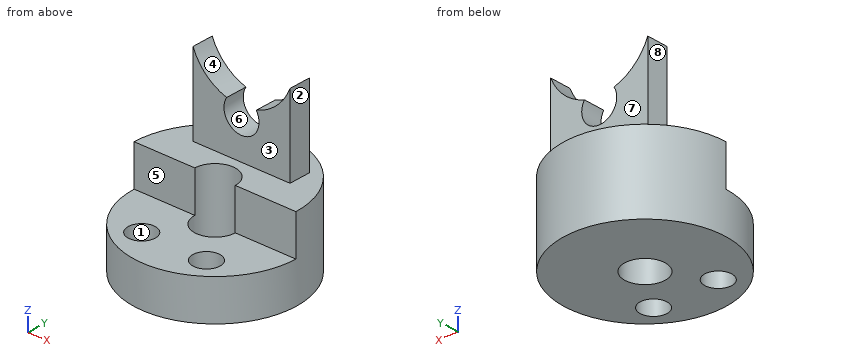
from build123d import *

# Parameters (mm, degrees)
SKETCH_1_R          = 30
EXTRUDE_1_DEPTH     = 15
EXTRUDE_2_DEPTH     = 15
SKETCH_3_R          = 7.5
CUT_EXTRUDE_1_DEPTH = 52.961524227
SKETCH_4_W          = 36
SKETCH_4_H          = 8
EXTRUDE_3_DEPTH     = 30
SKETCH_6_R          = 6.5
CUT_EXTRUDE_3_DEPTH = 79.619336044
SKETCH_5_R          = 19.313207916
CUT_EXTRUDE_4_DEPTH = 79.619336044
SKETCH_7_R          = 5
CUT_EXTRUDE_5_DEPTH = 62.846584384


with BuildPart() as part:
    # Эскиз1 → Бобышка-Вытянуть1 (new body)
    with BuildSketch(Plane.XY):
        Circle(SKETCH_1_R)
    extrude(amount=EXTRUDE_1_DEPTH)

    # Эскиз2 → Бобышка-Вытянуть2 (add)
    with BuildSketch(Plane.XY.offset(15)):
        with BuildLine():
            Line((-30, 0), (30, 0))
            ThreePointArc((30, 0), (0, 30), (-30, 0))
        make_face()
    extrude(amount=EXTRUDE_2_DEPTH)

    # Эскиз3 → Вырез-Вытянуть1 (cut, through all)
    with BuildSketch(Plane.XY.offset(30)):
        Circle(SKETCH_3_R)
    extrude(amount=-CUT_EXTRUDE_1_DEPTH, mode=Mode.SUBTRACT)

    # Эскиз4 → Бобышка-Вытянуть3 (add)
    with BuildSketch(Plane.XY.offset(30)):
        with Locations((0, 15)):
            Rectangle(SKETCH_4_W, SKETCH_4_H)
    extrude(amount=EXTRUDE_3_DEPTH)

    # Эскиз6 → Вырез-Вытянуть3 (cut, through all)
    with BuildSketch(Plane(origin=(0, 11, 0), x_dir=(-1, 0, 0), z_dir=(0, -1, 0))):
        with Locations(Location((0, -45, 0), (0, 0, 90))):
            Circle(SKETCH_6_R)
    extrude(amount=-CUT_EXTRUDE_3_DEPTH, mode=Mode.SUBTRACT)

    # Эскиз5 → Вырез-Вытянуть4 (cut, through all)
    with BuildSketch(Plane(origin=(0, 11, 0), x_dir=(-1, 0, 0), z_dir=(0, -1, 0))):
        with Locations((0, -67)):
            Circle(SKETCH_5_R)
    extrude(amount=-CUT_EXTRUDE_4_DEPTH, mode=Mode.SUBTRACT)

    # Эскиз7 → Вырез-Вытянуть5 (cut, through all)
    with BuildSketch(Plane.XY.offset(15)):
        with Locations((-12, -17)):
            Circle(SKETCH_7_R)
        with Locations((12, -17)):
            Circle(SKETCH_7_R)
    extrude(amount=-CUT_EXTRUDE_5_DEPTH, mode=Mode.SUBTRACT)


solid = part.part
CAD build for the part. Positions are in the model's coordinates, mm. Face numbers are marked on the shaded views. A direction names the side the tool comes from. Coordinates: 2 decimals unless noted, no trailing zeros. Write each loop counter-clockwise with the first axis right and the second up, starting at its lowest first coordinate (ties: lowest second). Pieces come first, ordered by that corner, then holes. Notation, with made-up numbers: M 70,-25.75 L 89,-25.75 A12 cw 89,-4.75 Z; hole C -35,-21 d4. An arc over 180 degrees is marked long. Return JSON: item names as keys, results as strings.
Item 1: Slice it at C-C, the plane x = -4. Write the cut outline in (y, z).
Findings below:
{"outline": "M -29.73,0 L -6.34,0 L -6.34,15 L -29.73,15 Z; M 6.34,0 L 29.73,0 L 29.73,30 L 19,30 L 19,39.88 L 11,39.88 L 11,30 L 6.34,30 Z"}
Item 2: Probe line 1 (Z direction, x = -3, y = -14); line 2 (Y direction, x = 17, z = 55.5); line 3 (Z direction, x = 0, y = 14). List the from-to ranges inside material, lowest first. Write a range as from..to.
Findings below:
{"line 1": "z = 0..15", "line 2": "y = 11..19", "line 3": "z = 0..38.5"}
Item 3: Which spindle directions (+Z, -Z, +X, -X, +Y, -Y) get a long thin tool onto all of the face, cutting with end or side? Do the marked faces 4, 5, 6, 7 and 8. Say none if no direction does.
Findings below:
{"face 4": "+Z, +Y, -Y", "face 5": "+Z, +X, -X, -Y", "face 6": "+Y, -Y", "face 7": "+Z, +X, -X, +Y", "face 8": "+Z, -X, +Y, -Y"}
Item 4: Slice it at D-D, the plane y = 12. Write the cut outline in (x, z), and give its area (3 significant figures).
Findings below:
{"outline": "M -27.5,0 L 27.5,0 L 27.5,30 L 18,30 L 18,60 A19.31 cw 5.49,48.48 A6.5 cw long -5.49,48.48 A19.31 cw -18,60 L -18,30 L -27.5,30 Z", "area": "2,300 mm2"}
Item 5: Slice it at A-A, the plane z = 45. Write the cut outline in (x, y).
Findings below:
{"outline": "M -18,11 L -6.5,11 L -6.5,19 L -18,19 Z; M 6.5,11 L 18,11 L 18,19 L 6.5,19 Z"}
Item 6: Drop flat-ended pins along their axis: pin 1 Ø24 at (x, z) = (-8, 37.5) entering from +Y; pin 2 Ø9 at (y, z) = (13.5, 51) entering from +X; pin 3 Ø1 at (x, z) = (-13.5, 22) entering from -Y; pin 4 Ø4 at (x, y) = (11.5, -19) entering from -Z. Give the stop position or say it passes through.
Findings below:
{"pin 1": "stops at y = 30", "pin 2": "stops at x = 18", "pin 3": "stops at y = 0", "pin 4": "passes through"}
Item 7: Slice it at B-B, the plane y = -15. Write the cut outline in (x, z).
Findings below:
{"outline": "M -25.98,0 L -16.58,0 L -16.58,15 L -25.98,15 Z; M -7.42,0 L 7.42,0 L 7.42,15 L -7.42,15 Z; M 16.58,0 L 25.98,0 L 25.98,15 L 16.58,15 Z"}
Item 8: Two-plate mould, pull along X, no slides. Class the marked faces 1, 2 and 3: +X half, -X half, draft (parallel to the pull), parting line (faces both ways), or undercut.
Findings below:
{"face 1": "undercut", "face 2": "+X half", "face 3": "draft"}
